Model file for the job. Use its own axes, mm. A direction names the side the tool comes from. Round coordinates to 2 decimals unless told otherwise and drop trailing zeros. Order: outer loops, then holes, each group sorted by start corner. A loop starts at its lowest first (then second) coordinate and runs counter-clockwise, first axis right, second up. Notation, with made-up numbers: (31, 84.5) - (62, 84.5) arc R22 cw to (62, 104.5) - close; hole circle Ø11 at (43, 21.25). An arc over 180 degrees is marked (long way). Answer as CSV lines item,"result". Start each with the question number.
1. 3-axis set-ups, long thin cutter, end or side, ignore diameter. For faces 1 (the face through (-52.9, 1.6, 31.3)), 2 (the face through (29.89, 1.57, 18.6)), 3 (the face through (67.802, 1.565, 18.905)): which of +Z, -Z, +X, -X, +Y, -Y reach the whole face in a straight line?
2. Pin check, flat tips, straight feed: pin 1 Ø1.6 at (x, y) = (9, 1.5) entering from -Z; pin 2 Ø1.6 at (x, y) = (-23, 2) entering from +Z; pin 3 Ø1 at (x, y) = (22.5, 0.5) entering from +Z. Stop position of each tip, or through.
3. Band-saw the part on A-A on x = -19.5. List the corners of the cut face in (y, z) (3 decimals), then the cut area to 3 significant figures.
4. Wall check: line 1 along X through (y, z) = (2.4, 11) (3 decimals); line 2 along Z through (x, y) = (22.5, 1.45); line 3 along X through (y, z) = (2.2, 2). Give the ranges that are in metal, low to high. Write a range as [from, to].
5. Band-saw the part on C-C on y = 2.3. State how many separate pieces and enclosed holes the cut face has, then the cut area to 3 significant figures.
6. Pull direction X, two halves, no side cores. Call faces 4 (the face through (1, 0, 15)), 5 (the face through (54.79, 1.57, 31.63)), 6 (the face through (-68.231, 1.565, 19.457)): released by +X, released by -X, zero draft, split by the parting line, or undercut.
7. Band-saw the part on B-B on z = 41.5. List the corners of the cut face in (x, y) (3 decimals), then the cut area to 3 significant figures.
8. Band-saw the part on D-D on x = 62. List the corners of the cut face in (y, z) (3 decimals).
```python
from build123d import *

# Parameters (mm, degrees)
BOSS_EXTRUDE1_DEPTH = 3.175


with BuildPart() as part:
    # Sketch2 → Boss-Extrude1 (new body)
    with BuildSketch(Plane(origin=(0, 0, 0), x_dir=(1, 0, 0), z_dir=(0, 1, 0))):
        with BuildLine():
            Line((1.5113, 0), (12.6238, 0))
            Line((12.6238, 0), (12.6238, 3.2512))
            Line((12.6238, 3.2512), (25.4762, 3.2512))
            Line((25.4762, 3.2512), (25.4762, 0))
            Line((25.4762, 0), (30.968022767, 0))
            ThreePointArc((30.968022767, 0), (31.727309935, -0.092126666), (32.442533737, -0.363160318))
            Line((32.442533737, -0.363160318), (104.164919451, -37.973926385))
            ThreePointArc((104.164919451, -37.973926385), (105.652252874, -41.929489283), (101.892440563, -43.858854449))
            Line((101.892440563, -43.858854449), (6.35, -19.05))
            Line((6.35, -19.05), (-6.35, -19.05))
            Line((-6.35, -19.05), (-100.721752751, -43.884671777))
            ThreePointArc((-100.721752751, -43.884671777), (-104.485708905, -41.973107934), (-103.023886624, -38.012739533))
            Line((-103.023886624, -38.012739533), (-32.450367647, -0.373529412))
            ThreePointArc((-32.450367647, -0.373529412), (-31.726300609, -0.094797562), (-30.95625, 0))
            Line((-30.95625, 0), (-25.4762, 0))
            Line((-25.4762, 0), (-25.4762, 3.2512))
            Line((-25.4762, 3.2512), (-12.6238, 3.2512))
            Line((-12.6238, 3.2512), (-12.6238, 0))
            Line((-12.6238, 0), (-1.5113, 0))
            Line((-1.5113, 0), (-1.5113, -9.4488))
            Line((-1.5113, -9.4488), (1.5113, -9.4488))
            Line((1.5113, -9.4488), (1.5113, 0))
        make_face()
        with BuildLine():
            Line((-52.083424577, -18.041159774), (-30.862867647, -6.723529412))
            ThreePointArc((-30.862867647, -6.723529412), (-30.138800609, -6.444797562), (-29.36875, -6.35))
            Line((-29.36875, -6.35), (-11.126341516, -6.35))
            ThreePointArc((-11.126341516, -6.35), (-8.876399737, -7.28482434), (-7.951371556, -9.538811345))
            Line((-7.951371556, -9.538811345), (-7.955433254, -10.472519677))
            ThreePointArc((-7.955433254, -10.472519677), (-8.620060106, -12.402622549), (-10.322386989, -13.529169988))
            Line((-10.322386989, -13.529169988), (-49.781290705, -23.913092018))
            ThreePointArc((-49.781290705, -23.913092018), (-53.545246858, -22.001528175), (-52.083424577, -18.041159774))
        make_face(mode=Mode.SUBTRACT)
        with BuildLine():
            Line((7.941592001, -9.529086738), (7.942778948, -10.451228904))
            ThreePointArc((7.942778948, -10.451228904), (8.607635671, -12.39131781), (10.3198084, -13.520230548))
            Line((10.3198084, -13.520230548), (50.025691322, -23.830386583))
            ThreePointArc((50.025691322, -23.830386583), (53.785503632, -21.901021417), (52.29817021, -17.945458519))
            Line((52.29817021, -17.945458519), (30.878579271, -6.713160318))
            ThreePointArc((30.878579271, -6.713160318), (30.163355469, -6.442126666), (29.404068301, -6.35))
            Line((29.404068301, -6.35), (11.116589371, -6.35))
            ThreePointArc((11.116589371, -6.35), (8.870080926, -7.281381315), (7.941592001, -9.529086738))
        make_face(mode=Mode.SUBTRACT)
    extrude(amount=BOSS_EXTRUDE1_DEPTH)


solid = part.part
```
Reply:
1,face 1,"+Z, +Y, -Y"
1,face 2,"+Y, -Y"
1,face 3,"-Z, +X, +Y, -Y"
2,pin 1,"stops at z = 0"
2,pin 2,"stops at z = 23.64"
2,pin 3,"stops at z = 23.37"
3,outline,"(0, -3.251) - (3.175, -3.251) - (3.175, 6.35) - (0, 6.35) - close; (0, 15.944) - (3.175, 15.944) - (3.175, 22.511) - (0, 22.511) - close"
3,area,"51.3 mm2"
4,line 1,"x = [-52.375, -38.881], [-8.002, 7.991], [39.053, 52.727]"
4,line 2,"z = [-3.25, 6.35], [16.68, 23.24]"
4,line 3,"x = [-35.5, -1.51], [1.51, 35.56]"
5,separate pieces,"1"
5,enclosed holes,"2"
5,area,"2,920 mm2"
6,face 4,"zero draft"
6,face 5,"undercut"
6,face 6,"released by -X"
7,outline,"(-104.63, 0) - (-91.66, 0) - (-91.66, 3.175) - (-104.63, 3.175) - close; (92.808, 0) - (105.784, 0) - (105.784, 3.175) - (92.808, 3.175) - close"
7,area,"82.4 mm2"
8,outline,"(0, 15.863) - (3.175, 15.863) - (3.175, 33.5) - (0, 33.5) - close"
